Here's how the part is built. I have some questions about the finished solid (model axes, mm). Coordinates: 2 decimals unless noted, no trailing zeros.
```python
from build123d import *

# Parameters (mm, degrees)
F0_R     = 3
F0_R_2   = 2.5
F1_DEPTH = 578
F2_R     = 2
F3_R     = 7


# Not quite as in the source:
# - a feature names something its author has since deleted; it is built from what else it names


with BuildPart() as f1:
    # F0 (on Top) → F1 (new body)
    with BuildSketch(Plane.XY):
        with BuildLine():
            Line((18.15, -15), (30, -15))
            Line((30, -15), (30, -3.15))
            Line((30, -3.15), (27.5, -3.15))
            Line((27.5, -3.15), (27.5, -5.15))
            Line((27.5, -5.15), (21.5477069044, -5.15))
            ThreePointArc((21.5477069044, -5.15), (19.5, 0), (21.5477069044, 5.15))
            Line((21.5477069044, 5.15), (27.5, 5.15))
            Line((27.5, 5.15), (27.5, 3.15))
            Line((27.5, 3.15), (30, 3.15))
            Line((30, 3.15), (30, 15))
            Line((30, 15), (18.15, 15))
            Line((18.15, 15), (18.15, 12.5))
            Line((18.15, 12.5), (20.15, 12.5))
            Line((20.15, 12.5), (20.15, 6.5477069044))
            ThreePointArc((20.15, 6.5477069044), (15, 4.5), (9.85, 6.5477069044))
            Line((9.85, 6.5477069044), (9.85, 12.5))
            Line((9.85, 12.5), (11.85, 12.5))
            Line((11.85, 12.5), (11.85, 15))
            Line((11.85, 15), (-11.85, 15))
            Line((-11.85, 15), (-11.85, 12.5))
            Line((-11.85, 12.5), (-9.85, 12.5))
            Line((-9.85, 12.5), (-9.85, 6.5477069044))
            ThreePointArc((-9.85, 6.5477069044), (-15, 4.5), (-20.15, 6.5477069044))
            Line((-20.15, 6.5477069044), (-20.15, 12.5))
            Line((-20.15, 12.5), (-18.15, 12.5))
            Line((-18.15, 12.5), (-18.15, 15))
            Line((-18.15, 15), (-30, 15))
            Line((-30, 15), (-30, 3.15))
            Line((-30, 3.15), (-27.5, 3.15))
            Line((-27.5, 3.15), (-27.5, 5.15))
            Line((-27.5, 5.15), (-21.5477069044, 5.15))
            ThreePointArc((-21.5477069044, 5.15), (-19.5, 0), (-21.5477069044, -5.15))
            Line((-21.5477069044, -5.15), (-27.5, -5.15))
            Line((-27.5, -5.15), (-27.5, -3.15))
            Line((-27.5, -3.15), (-30, -3.15))
            Line((-30, -3.15), (-30, -15))
            Line((-30, -15), (-18.15, -15))
            Line((-18.15, -15), (-18.15, -12.5))
            Line((-18.15, -12.5), (-20.15, -12.5))
            Line((-20.15, -12.5), (-20.15, -6.5477069044))
            ThreePointArc((-20.15, -6.5477069044), (-15, -4.5), (-9.85, -6.5477069044))
            Line((-9.85, -6.5477069044), (-9.85, -12.5))
            Line((-9.85, -12.5), (-11.85, -12.5))
            Line((-11.85, -12.5), (-11.85, -15))
            Line((-11.85, -15), (11.85, -15))
            Line((11.85, -15), (11.85, -12.5))
            Line((11.85, -12.5), (9.85, -12.5))
            Line((9.85, -12.5), (9.85, -6.5477069044))
            ThreePointArc((9.85, -6.5477069044), (15, -4.5), (20.15, -6.5477069044))
            Line((20.15, -6.5477069044), (20.15, -12.5))
            Line((20.15, -12.5), (18.15, -12.5))
            Line((18.15, -12.5), (18.15, -15))
        make_face()
        with Locations((-25, -10)):
            Circle(F0_R, mode=Mode.SUBTRACT)
        with Locations((25, -10)):
            Circle(F0_R, mode=Mode.SUBTRACT)
        with Locations((-15, 0)):
            Circle(F0_R_2, mode=Mode.SUBTRACT)
        with Locations((-25, 10)):
            Circle(F0_R, mode=Mode.SUBTRACT)
        Polygon((-7, 7), (-7, 12.5), (0, 12.5), (7, 12.5), (7, 7), (10, 0), (7, -7), (7, -12.5), (0, -12.5), (-7, -12.5), (-7, -7), (-10, 0), align=None, mode=Mode.SUBTRACT)
        with Locations((15, 0)):
            Circle(F0_R_2, mode=Mode.SUBTRACT)
        with Locations((25, 10)):
            Circle(F0_R, mode=Mode.SUBTRACT)
    extrude(amount=F1_DEPTH)

    # F2
    f2_edges = [f1.edges().sort_by_distance(p)[0] for p in [
        (-7, 12.5, 289),
        (7, 12.5, 289),
    ]]
    fillet(f2_edges, radius=F2_R)

    # F3
    f3_edges = [f1.edges().sort_by_distance(p)[0] for p in [
        (-7, 7, 289),
        (-10, 0, 289),
        (7, 7, 289),
        (10, 0, 289),
    ]]
    fillet(f3_edges, radius=F3_R)


solid = f1.part
```
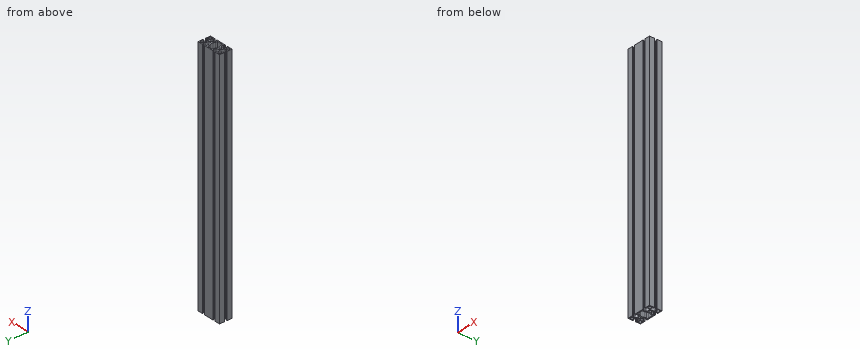
Q1. I need wall thicknesses on L1, parallel to Y at x = 25, z = 118; L2, parallel to X at y = -10.5, z = 538.5; L3, parallel to Y at x = -2.5, z = 431. Which ranges of each line are inside material? Lowest first, please.
Q2. If we section it at A-A on z = 157: Give the number of separate pieces and of enclosed holes in the cut face, then the cut area to 3 significant figures.
Q3. Will these pins go through, and if not, where does the flat tip stop? pin 1 (6 mm diameter, centred on x = 15, z = 94, fed in from +Y); pin 2 (6 mm diameter, centred on x = -15, y = 0, fed in from +Z); pin 3 (2 mm diameter, centred on y = 1.5, z = 401.5, fed in from +X).
Reply:
1. L1: y = -15 to -13, -7 to -5.15, 5.15 to 7, 13 to 15
1. L2: x = -30 to -27.96, -22.04 to -20.15, -9.85 to -7, 7 to 9.85, 20.15 to 22.04, 27.96 to 30
1. L3: y = -15 to -12.5, 12.5 to 15
2. separate pieces: 1
2. enclosed holes: 7
2. area: 710 mm2
3. pin 1: stops at y = 5.13
3. pin 2: stops at z = 578
3. pin 3: stops at x = 19.93
